Here's how the part is built. I have some questions about the finished solid (model axes, mm). A direction names the side the tool comes from. Coordinates: 2 decimals unless noted, no trailing zeros. Write each loop counter-clockwise with the first axis right and the second up, starting at its lowest first coordinate (ties: lowest second). Pieces come first, ordered by that corner, then holes.
(1) Imagine slicing it at B-B, the plane z = 0.65. List the corners of the cut face in (x, y) for me.
(2) For pin 1 Ø1.5 at (x, z) = (-3, 2) entering from +Y, with a flat end and sliding along its axis, tell me the tip position at first contact or that it passes through.
(3) Which directions (+Z, -Z, +X, -X, +Y, -Y) give clear straight access to the entire face, cutting with the end or side of a thin tool? Please do faces 1 (the flat face through (-1, -5, 0)), 2 (the cylindrical face through (1.8, -7.176, 1.972)).
(4) Thinking about a two-plate mould opening in X: for faces 3 (the flat face through (-5.3, -6, 2)), 4 (the flat face through (5.3, -4, 2)), 5 (the flat face through (-4, -11.3, 2)), 6 (the cylindrical face through (-2.43, 2.23, 1.98)), which applies, released by +X, released by -X, zero draft, split by the parting line, or undercut?
(5) Imagine slicing it at C-C, the plane x = 4.5. List the corners of the cut face in (y, z) for me.
(6) Imagine slicing it at D-D, the plane z = 3. List the corners of the cut face in (x, y) for me.
(7) Please list where these lines run through material, in increasing order: probe 1 along Y at (x, z) = (0, 2.15); probe 2 along Y at (x, z) = (-0.75, 2.85); probe 3 along X at (y, z) = (-7.75, 2.2).
(8) Imagine slicing it at A-A, the plane x = 0. List the corners of the cut face in (y, z) for me.
```python
from build123d import *

# Parameters (mm, degrees)
F0_R     = 3.3
F1_DEPTH = 4
F2_W     = 3.5
F2_H     = 4
F3_DEPTH = 4
F4_SIZE  = 0.4
F5_R     = 16.2
F6_DEPTH = 7.1


with BuildPart() as f1:
    # F0 (on Top) → F1 (new body)
    with BuildSketch(Plane.XY):
        with BuildLine():
            ThreePointArc((-5.3, 0), (0, -5.3), (5.3, 0))
            ThreePointArc((5.3, 0), (0, 5.3), (-5.3, 0))
        make_face()
        Circle(F0_R, mode=Mode.SUBTRACT)
        with BuildLine():
            Line((5.3, -7.3), (5.3, 0))
            ThreePointArc((5.3, 0), (0, -5.3), (-5.3, 0))
            Line((-5.3, 0), (-5.3, -7.3))
            Line((-5.3, -7.3), (5.3, -7.3))
        make_face()
    extrude(amount=F1_DEPTH)

    # F2 (on face) → F3 (join)
    with BuildSketch(Plane.XZ.offset(7.3)):
        with Locations((-3.55, 2)):
            Rectangle(F2_W, F2_H)
    extrude(amount=F3_DEPTH)

    # F4
    f4_edges = [f1.edges().sort_by_distance(p)[0] for p in [
        (-3.3, 0, 4),
        (-3.3, 0, 0),
    ]]
    chamfer(f4_edges, length=F4_SIZE)

    # F5 (on face) → F6 (cut, through all)
    with BuildSketch(Plane.YZ.offset(5.3)):
        with Locations((-23.376069, 2)):
            Circle(F5_R)
    extrude(amount=-F6_DEPTH, mode=Mode.SUBTRACT)


solid = f1.part
```
Recorded:
1. outline: (-5.3, -11.3) - (-1.8, -11.3) - (-1.8, -7.23) - (5.3, -7.23) - (5.3, 0) arc R5.3 ccw to (-5.3, 0) - close; hole circle Ø6.6 at (0, 0)
2. pin 1: stops at y = 4.8
3. face 1: -Z, +X, -X, +Y, -Y
3. face 2: +X, -Y
4. face 3: released by -X
4. face 4: released by +X
4. face 5: zero draft
4. face 6: undercut
5. outline: (-7.3, 0) - (2.8, 0) - (2.8, 4) - (-7.3, 4) arc R16.2 cw to start
6. outline: (-5.3, -11.3) - (-1.8, -11.3) - (-1.8, -7.21) - (5.3, -7.21) - (5.3, 0) arc R5.3 ccw to (-5.3, 0) - close; hole circle Ø6.6 at (0, 0)
7. probe 1: y = -7.18 to -3.3, 3.3 to 5.3
7. probe 2: y = -7.2 to -3.21, 3.21 to 5.25
7. probe 3: x = -5.3 to -1.8
8. outline: (-7.3, 0) - (-3.7, 0) - (-3.3, 0.4) - (-3.3, 3.6) - (-3.7, 4) - (-7.3, 4) arc R16.2 cw to start; (3.3, 0.4) - (3.7, 0) - (5.3, 0) - (5.3, 4) - (3.7, 4) - (3.3, 3.6) - close
